Part model, mm, in its own coordinate system. A direction names the side the tool comes from. Round coordinates to 2 decimals unless told otherwise and drop trailing zeros. Loops run counter-clockwise (first coordinate to the right, second up) from the corner with the lowest first, then second, coordinate; pieces in that order, holes last.
(1) Cut at A-A on y = 97.5. List the corners of the cut face in (x, z).
(2) Flat gauge pins, fed straight in: pin 1 (10 mm diameter, centred on x = 7.5, y = 61.5, fed in from -Z); pin 2 (10 mm diameter, centred on x = 12.5, y = 14, fed in from -Z); pin 3 (2.5 mm diameter, centred on x = 4, y = 97.5, fed in from -Z); pin 4 (2 mm diameter, centred on x = 15, z = -11, fed in from -Y). Where does each tip first touch, or does it go through?
(3) Mould opens along X. For faces 1 (the face through (4, 96, -48)), 2 (the face through (20, 50, -3)), 3 (the face through (9.86, 44.87, -0.39)) say: +X half, -X half, draft (parallel to the pull), parting line (faces both ways), or undercut.
(4) Cut at B-B on x = 10. List the corners of the cut face in (y, z), then the cut area to 3 significant figures.
(5) Probe probe 1 along Y at (x, z) = (10, 1.75); probe 2 along X at (y, z) = (97.5, -47.7); probe 3 along X at (y, z) = (97, -48). List the from-to ranges inside material, lowest first.
(6) Cut at D-D on x = 16. List the corners of the cut face in (y, z), then the cut area to 3 significant figures.
(7) Cut at C-C on y = 32.5. List the corners of the cut face in (x, z), then the cut area to 3 significant figures.
(8) Tool access for faces 4 (the face through (10, 50, 4)), 5 (the face through (10, 21, 0)), 6 (the face through (9.566, 30.548, 3.131)): list every direction of +Z, -Z, +X, -X, +Y, -Y with a clear straight run to the whole face (end or side of a thin tool).
from build123d import *

# Parameters (mm, degrees)
SKETCH1_W           = 20
SKETCH1_H           = 40
SKETCH1_R           = 2
BOSS_EXTRUDE1_DEPTH = 6.35
SKETCH2_W           = 20
SKETCH2_H           = 6.35
BOSS_EXTRUDE2_DEPTH = 10
BOSS_EXTRUDE3_DEPTH = 20
SKETCH4_R           = 1.5
CUT_EXTRUDE1_DEPTH  = 23.2
FILLET1_R           = 5


with BuildPart() as part:
    # Sketch1 → Boss-Extrude1 (new body)
    with BuildSketch(Plane.XY):
        with Locations((10, 20)):
            Rectangle(SKETCH1_W, SKETCH1_H)
        with Locations((10, 32.5)):
            Circle(SKETCH1_R, mode=Mode.SUBTRACT)
        with Locations((10, 7.5)):
            Circle(SKETCH1_R, mode=Mode.SUBTRACT)
    extrude(amount=BOSS_EXTRUDE1_DEPTH)

    # Sketch2 → Boss-Extrude2 (add)
    with BuildSketch(Plane(origin=(0, 40, 0), x_dir=(1, 0, 0), z_dir=(0, 1, 0))):
        with Locations((10, -3.175)):
            Rectangle(SKETCH2_W, SKETCH2_H)
    extrude(amount=BOSS_EXTRUDE2_DEPTH)

    # Sketch3 → Boss-Extrude3 (add)
    with BuildSketch(Plane(origin=(20, 0, 0), x_dir=(0, 0, -1), z_dir=(1, 0, 0))):
        Polygon((50, 100), (50, 95), (0, 45), (0, 50), align=None)
    extrude(amount=-BOSS_EXTRUDE3_DEPTH)

    # Sketch4 → Cut-Extrude1 (cut)
    with BuildSketch(Plane(origin=(0, 0, -50), x_dir=(-1, 0, 0), z_dir=(0, 0, -1))):
        with Locations((-16, 97.5)):
            Circle(SKETCH4_R)
        with Locations((-4, 97.5)):
            Circle(SKETCH4_R)
    extrude(amount=-CUT_EXTRUDE1_DEPTH, mode=Mode.SUBTRACT)

    # Fillet1
    fillet1_edges = [part.edges().sort_by_distance(p)[0] for p in [
        (10, 50, 0),
        (10, 45, 0),
    ]]
    fillet(fillet1_edges, radius=FILLET1_R)


solid = part.part
Final values:
1. outline: (0, -50) - (2.5, -50) - (2.5, -47.5) - (0, -47.5) - close; (5.5, -50) - (14.5, -50) - (14.5, -47.5) - (5.5, -47.5) - close; (17.5, -50) - (20, -50) - (20, -47.5) - (17.5, -47.5) - close
2. pin 1: stops at z = -21.5
2. pin 2: stops at z = 0
2. pin 3: passes through
2. pin 4: stops at y = 55
3. face 1: undercut
3. face 2: +X half
3. face 3: draft
4. outline: (0, 0) - (5.5, 0) - (5.5, 6.35) - (0, 6.35) - close; (9.5, 0) - (30.5, 0) - (30.5, 6.35) - (9.5, 6.35) - close; (34.5, 0) - (42.93, 0) arc R5 cw to (46.46, -1.46) - (95, -50) - (100, -50) - (51.46, -1.46) arc R5 cw to (50, 2.07) - (50, 6.35) - (34.5, 6.35) - close
4. area: 518 mm2
5. probe 1: y = 0 to 5.5, 9.5 to 30.5, 34.5 to 50.01
5. probe 2: x = 0 to 2.5, 5.5 to 14.5, 17.5 to 20
5. probe 3: x = 0 to 2.59, 5.41 to 14.59, 17.41 to 20
6. outline: (0, 0) - (42.93, 0) arc R5 cw to (46.46, -1.46) - (95, -50) - (96, -50) - (96, -46) - (51.46, -1.46) arc R5 cw to (50, 2.07) - (50, 6.35) - (0, 6.35) - close; (99, -50) - (100, -50) - (99, -49) - close
6. area: 561 mm2
7. outline: (0, 0) - (8, 0) - (8, 6.35) - (0, 6.35) - close; (12, 0) - (20, 0) - (20, 6.35) - (12, 6.35) - close
7. area: 102 mm2
8. face 4: +Z, +X, -X, +Y
8. face 5: -Z, +X, -X, -Y
8. face 6: +Z, -Z
